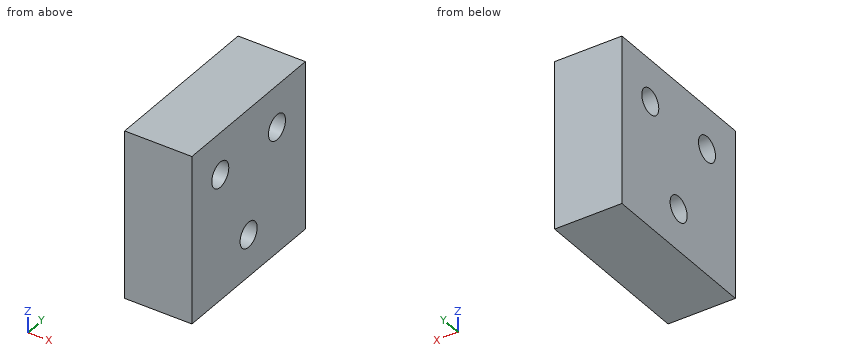
Autodesk Inventor part; units mm, degrees
ref_plane "YZ Plane" through (0, 0, 0) normal (1, 0, 0) x (0, 1, 0)
ref_plane "XZ Plane" through (0, 0, 0) normal (0, 1, 0) x (-1, 0, 0)
ref_plane "XY Plane" through (0, 0, 0) normal (0, 0, 1) x (1, 0, 0)
sketch "Sketch1" plane through (0, 0, 0) normal (1, 0, 0) x (0, 1, 0)
  line L0 (15.8212, 35.7681) -> (-9.5788, 35.7681)
  line L1 (-9.5788, 35.7681) -> (-9.5788, 10.3681)
  line L2 (-9.5788, 10.3681) -> (15.8212, 10.3681)
  line L3 (15.8212, 10.3681) -> (15.8212, 35.7681)
  point P0 (0, 0)
  dimension "d0" = 25.4
  dimension "d1" = 25.4
extrude "Extrusion1" add sketch "Sketch1" along normal blind 10.16
sketch "Sketch2" plane through (10.16, 0, 0) normal (1, 0, 0) x (0, 0, -1)
  line L0 (-35.7681, 15.8212) -> (-35.7681, -9.5788)
  line L1 (-10.3681, 15.8212) -> (-35.7681, 15.8212)
  line L2 (-35.7681, -9.5788) -> (-10.3681, -9.5788)
  point P0 (0, 0)
  point P1 (-29.4181, 9.4712)
  point P2 (-29.4181, -3.2288)
  point P3 (-16.7181, 3.1212)
  dimension "d4" = 19.05
  dimension "d5" = 12.7
  dimension "d6" = 6.35
  dimension "d7" = 6.35
  dimension "d8" = 0
  dimension "d9" = 6.35
hole "Hole1" at (10.16, 9.4712, 29.4181) at (10.16, -3.2288, 29.4181) at (10.16, 3.1212, 16.7181) direction (-1, 0, 0) diameter 3.81 depth 10.9728 tip angle 118.188
properties part number "tOPgRIPPERcLAMP"
Geometry: final body of the model. Coordinates: model frame, mm. Give positions to 0.01 mm unless a question says otherwise; leave off trailing zeros. Order: outer loops, then holes, each group sorted by start corner. A loop starts at its lowest first (then second) coordinate and runs counter-clockwise, first axis right, second up. Notation, with made-up numbers: (45, 20.5) -> (56, 20.5) arc R14 ccw to (56, 31.5) -> close; hole circle Ø1 at (-8.5, -37.5). An arc over 180 degrees is marked (long way). Write each question's results on one line, items separated by ' | '. Start each with the question number.
1) Section A-A (y = -2). Return loops of the section in (x, z), then the cut area to 3 significant figures.
2) First-contact query: pin 1 (3 mm diameter, centred on y = 3.12, z = 16.72, fed in from -X); pin 2 (1 mm diameter, centred on y = -5.5, z = 28.5, fed in from -X). Flat tips, straight axial feed; report the tip coordinate or a pass-through.
3) Section B-B (x = 8.25). Return loops of the section in (y, z) (3 decimals).
4) Line query: line 1 (Y direction, x = 3, z = 30); line 2 (Y direction, x = 8.25, z = 30.75); line 3 (Y direction, x = 8, z = 15.5). Output: solid intervals per line, ascending. Write a range as from..to.
5) Section C-C (z = 16.5). Return loops of the section in (x, y).
Calculated:
1) outline: (0, 10.37) -> (10.16, 10.37) -> (10.16, 27.96) -> (0, 27.96) -> close; (0, 30.87) -> (10.16, 30.87) -> (10.16, 35.77) -> (0, 35.77) -> close | area: 228 mm2
2) pin 1: through | pin 2: x = 0
3) outline: (-9.579, 10.368) -> (15.821, 10.368) -> (15.821, 35.768) -> (-9.579, 35.768) -> close; hole circle Ø3.81 at (-3.229, 29.418); hole circle Ø3.81 at (3.121, 16.718); hole circle Ø3.81 at (9.471, 29.418)
4) line 1: -9.58..-5.04, -1.41..7.66, 11.29..15.82 | line 2: -9.58..-4.59, -1.87..8.11, 10.83..15.82 | line 3: -9.58..1.66, 4.59..15.82
5) outline: (0, -9.58) -> (10.16, -9.58) -> (10.16, 1.23) -> (0, 1.23) -> close; (0, 5.01) -> (10.16, 5.01) -> (10.16, 15.82) -> (0, 15.82) -> close
